Design review of the part built by this model. Coordinates are the model's own, in mm. Give positions to 0.01 mm unless a question says otherwise; leave off trailing zeros. Loops run counter-clockwise (first coordinate to the right, second up) from the corner with the lowest first, then second, coordinate; pieces in that order, holes last. Notation, with made-up numbers: M 24,43.25 L 62,43.25 A14 cw 62,52.25 Z; hole C -21.5,51 d8. An arc over 180 degrees is marked long. Use CSV: the item, a comma, the result in double quotes.
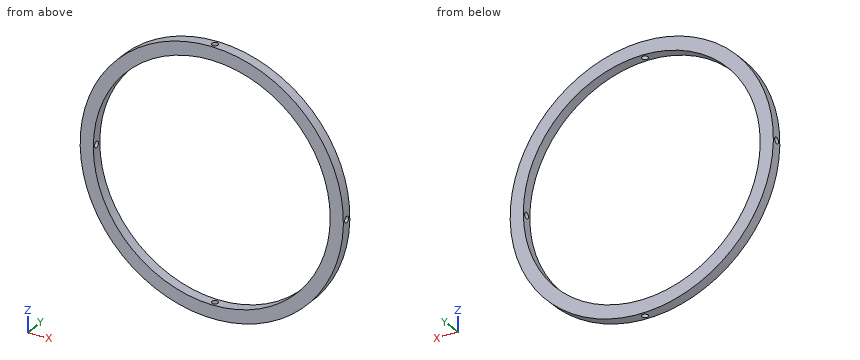
from build123d import *

# Parameters (mm, degrees)
OUTER_RING_MAIN_SKETCH_R   = 63.5
OUTER_RING_MAIN_BODY_DEPTH = 5
CENTER_HOLE_SKETCH_R       = 57.15
CENTER_HOLE_DEPTH          = 90.94164775
PIN_HOLE_DEPTH             = 90.94164775
PIN_HOLE_DEPTH_BACK        = 90.94164775
PIN_HOLE_SKETCH_R          = 1.5
PIN_HOLE_2_DEPTH           = 90.941647898
PIN_HOLE_2_DEPTH_BACK      = 90.941647898
PIN_HOLE_2_SKETCH_R        = 1.5


with BuildPart() as part:
    # Outer Ring Main Sketch → Outer Ring Main Body (new body)
    with BuildSketch(Plane(origin=(0, 0, 0), x_dir=(1, 0, 0), z_dir=(0, 1, 0))):
        with Locations(Location((0, 0, 0), (0, 0, 270))):
            Circle(OUTER_RING_MAIN_SKETCH_R)
    extrude(amount=OUTER_RING_MAIN_BODY_DEPTH)

    # Center Hole Sketch → Center Hole (cut, through all)
    with BuildSketch(Plane.XZ):
        with Locations(Location((0, 0, 0), (0, 0, 270))):
            Circle(CENTER_HOLE_SKETCH_R)
    extrude(amount=-CENTER_HOLE_DEPTH, mode=Mode.SUBTRACT)

    # Pin Hole Sketch → Pin Hole (cut, two sides: drawn at the far end of the back side and taken through both)
    with BuildSketch(Plane.XY.offset(-PIN_HOLE_DEPTH_BACK)):
        with Locations((0, 2.5)):
            Circle(PIN_HOLE_SKETCH_R)
    extrude(amount=PIN_HOLE_DEPTH + PIN_HOLE_DEPTH_BACK, mode=Mode.SUBTRACT)

    # Pin Hole 2 Sketch → Pin Hole 2 (cut, two sides: drawn at the far end of the back side and taken through both)
    with BuildSketch(Plane(origin=(0, 0, 0), x_dir=(0, 0, -1), z_dir=(1, 0, 0)).offset(-PIN_HOLE_2_DEPTH_BACK)):
        with Locations((0, 2.5)):
            Circle(PIN_HOLE_2_SKETCH_R)
    extrude(amount=PIN_HOLE_2_DEPTH + PIN_HOLE_2_DEPTH_BACK, mode=Mode.SUBTRACT)


solid = part.part
(1) We need section A-A on z = 0. State the section outline as (x, y) points.
A:
outline,"M -63.5,0 L -57.15,0 L -57.15,1 L -63.5,1 Z; M -63.5,4 L -57.15,4 L -57.15,5 L -63.5,5 Z; M 57.15,0 L 63.5,0 L 63.5,1 L 57.15,1 Z; M 57.15,4 L 63.5,4 L 63.5,5 L 57.15,5 Z"
(2) Wall thickness on line 1 along Y through (x, z) = (0, 59); line 2 along Z through (x, y) = (-15.5, 2); line 3 along Z through (x, y) = (-21.5, 2.5): over which ranges is each line inside the solid? List them lowest first. Write a range as [from, to].
A:
line 1,"[0, 1], [4, 5]"
line 2,"[-61.58, -55.01], [55.01, 61.58]"
line 3,"[-59.75, -52.95], [52.95, 59.75]"
(3) We need section B-B on x = 3. State the section outline as (y, z) points, then the cut area to 3 significant figures.
A:
outline,"M 0,-63.43 L 5,-63.43 L 5,-57.07 L 0,-57.07 Z; M 0,57.07 L 5,57.07 L 5,63.43 L 0,63.43 Z"
area,"63.6 mm²"
(4) We need section C-C on z = 42. State the section outline as (x, y) points.
A:
outline,"M -47.63,0 L -38.76,0 L -38.76,5 L -47.63,5 Z; M 38.76,0 L 47.63,0 L 47.63,5 L 38.76,5 Z"
(5) We need section D-D on y = 2.5. State the section outline as (x, z) points, then the cut area to 3 significant figures.
A:
outline,"M -63.48,-1.5 A63.5 ccw -1.5,-63.48 L -1.5,-57.13 A57.15 cw -57.13,-1.5 Z; M -63.48,1.5 L -57.13,1.5 A57.15 cw -1.5,57.13 L -1.5,63.48 A63.5 ccw Z; M 1.5,-63.48 A63.5 ccw 63.48,-1.5 L 57.13,-1.5 A57.15 cw 1.5,-57.13 Z; M 1.5,57.13 A57.15 cw 57.13,1.5 L 63.48,1.5 A63.5 ccw 1.5,63.48 Z"
area,"2,330 mm²"
(6) Clearance check with flat-ended pins moving along their axes: P1, Ø2, axis at y = 2, z = 13.5, coming from the -X side; P2, Ø3, axis at y = 2, z = 46.5, coming from the +X side. State where each tip first meets the part, or that it passes through.
A:
P1,"x = -62.26"
P2,"x = 44.8"
